```python
from build123d import *

# Parameters (mm, degrees)
SKETCH_2_R        = 9.874937623
EXTRUDE_1_DEPTH   = 40
SKETCH_2_R_2      = 10.181689967
EXTRUDE_1_2_DEPTH = 40
EXTRUDE_1_3_DEPTH = 40
EXTRUDE_5_DEPTH   = 40
EXTRUDE_2_DEPTH   = 4


# Read off the part's stored shape, not the designer's step: 拉伸-薄壁1
with BuildPart() as part:
    # 草图2 → Extrude 1 (new body)
    with BuildSketch(Plane(origin=(0, 140, 0), x_dir=(1, 0, 0), z_dir=(0, 1, 0))):
        with Locations(Location((-234.331213423, -10.749627478, 0), (0, 0, 270))):
            Circle(SKETCH_2_R)
    extrude_1 = extrude(amount=EXTRUDE_1_DEPTH)



with BuildPart() as body_2:
    # 草图2 → Extrude 1 2 (new body)
    with BuildSketch(Plane(origin=(0, 140, 0), x_dir=(1, 0, 0), z_dir=(0, 1, 0))):
        with Locations(Location((253.431386216, -10.749627478, 0), (0, 0, 270))):
            Circle(SKETCH_2_R_2)
    extrude_1_2 = extrude(amount=EXTRUDE_1_2_DEPTH)


with BuildPart() as part_1:
    add(part.part)

    add(body_2.part)  # Extrude 1 3 merges body 2
    # Extrude 1 3 outline → Extrude 1 3 (add)
    with BuildSketch(Plane.XY):
        with BuildLine():
            Line((-360, -135), (-350, -135))
            Line((-350, -135), (-335, -150))
            Line((-335, -150), (335, -150))
            ThreePointArc((335, -150), (345.606601718, -145.606601718), (350, -135))
            Line((350, -135), (350, 135))
            ThreePointArc((350, 135), (345.606601718, 145.606601718), (335, 150))
            Line((335, 150), (-335, 150))
            Line((-335, 150), (-335, 140))
            Line((-335, 140), (335, 140))
            ThreePointArc((335, 140), (338.535533906, 138.535533906), (340, 135))
            Line((340, 135), (340, -135))
            ThreePointArc((340, -135), (338.535533906, -138.535533906), (335, -140))
            Line((335, -140), (-330.857864376, -140))
            Line((-330.857864376, -140), (-341.617461171, -129.240403205))
            ThreePointArc((-341.617461171, -129.240403205), (-345.993586414, -118.835156387), (-350, -108.282039139))
            Line((-350, -108.282039139), (-350, 108.282039139))
            ThreePointArc((-350, 108.282039139), (-345.653254032, 119.682560505), (-340.875063682, 130.909090909))
            Line((-340.875063682, 130.909090909), (-350, 135))
            Line((-350, 135), (-360, 135))
            Line((-360, 135), (-360, 110.011554075))
            ThreePointArc((-360, 110.011554075), (-378.877101502, 0), (-360, -110.011554075))
            Line((-360, -110.011554075), (-360, -135))
        make_face()
        with BuildLine():
            Line((-360, 74.850130461), (-360, -74.850130461))
            ThreePointArc((-360, -74.850130461), (-368.877101502, 0), (-360, 74.850130461))
        make_face(mode=Mode.SUBTRACT)
    extrude(amount=EXTRUDE_1_3_DEPTH)

    # 镜向3: Extrude 1, Extrude 1 2 across plane
    add(extrude_1.mirror(Plane.ZX))
    add(extrude_1_2.mirror(Plane.ZX))

    # 草图1<3> → 拉伸-薄壁5 (add)
    with BuildSketch(Plane.XY):
        Polygon((-350, 135), (-335, 150), (-327.928932188, 142.928932188), (-342.928932188, 127.928932188), align=None)
    extrude(amount=EXTRUDE_5_DEPTH)

    # 草图1<4> → 凸台-拉伸2 (add)
    with BuildSketch(Plane.XY):
        with BuildLine():
            Line((-335, -150), (335, -150))
            ThreePointArc((335, -150), (345.606601718, -145.606601718), (350, -135))
            Line((350, -135), (350, 135))
            ThreePointArc((350, 135), (345.606601718, 145.606601718), (335, 150))
            Line((335, 150), (-335, 150))
            Line((-335, 150), (-350, 135))
            Line((-350, 135), (-350, -135))
            Line((-350, -135), (-335, -150))
        make_face()
    extrude(amount=EXTRUDE_2_DEPTH)


solid = part_1.part
```
For this review, take the finished solid that the model builds, in its own axes (mm). A direction names the side the tool comes from. Coordinates: 2 decimals unless noted, no trailing zeros. Order: outer loops, then holes, each group sorted by start corner. A loop starts at its lowest first (then second) coordinate and runs counter-clockwise, first axis right, second up. Notation, with made-up numbers: (76.5, -19.5) - (105.5, -19.5) arc R24 cw to (105.5, -5.5) - close; hole circle Ø5 at (-24.75, -2). An arc over 180 degrees is marked (long way). Answer as a JSON object with one key per item and string values. Group by question number.
1. We need section D-D on z = 10. Give the number of separate pieces and of enclosed holes in the cut face, then the cut area to 3 significant figures.
2. We need section A-A on y = 18. State the section outline as (x, z) points.
3. The part is to be moulded in two halves that separate along Y. For faces 4 (the flat face through (-10, 2, 4)), 5 (the cylindrical face through (243.5, 164.8, 8.5)), 6 (the flat face through (-343, -142, 20)), say which applies: pulls with the +Y half, pulls with the -Y half, needs draft (parallel to the pull), parting line crosses it, or undercut.
4. We need section C-C on y = -67. State the section outline as (x, z) points.
5. We need section B-B on x = -101. State the section outline as (y, z) points, then the cut area to 3 significant figures.
6. Clearance check with flat-ended pins moving along their axes: P1, Ø8, axis at x = -356.5, z = 26, coming from the -Y side; P2, Ø5, axis at x = 241.5, y = -123.5, coming from the +Z side; P3, Ø18, axis at x = 50, z = 31, coming from the +Y side; P4, Ø4, axis at x = 29, y = 120, coming from the -Z side. State where each tip first meets the part, or that it passes through.
7. For faces 1 (the cylindrical face through (-243.97, -164.79, 8.61)), 2 (the cylindrical face through (-345.935, -118.982, 21.748)), 3 (the flat face through (254, -180, 11)), list the 3-axis set-ups (+Z, -Z, +X, -X, +Y, -Y) from which the entire face can be reached by the end or side of a thin tool; tool diameter is ignored.
8. For probe 1 along X at (y, z) = (80, 20.5); probe 2 along Y at (x, z) = (-64, 14); probe 3 along X at (y, z) = (-56.5, 20), list the stretches that pass through material, from the lowest coordinate up.
Final values:
{
 "1": {"separate pieces": "1", "enclosed holes": "2", "area": "24,000 mm²"},
 "2": {"outline": "(-378.39, 0) - (-368.37, 0) - (-368.37, 40) - (-378.39, 40) - close; (-360, 0) - (350, 0) - (350, 40) - (340, 40) - (340, 4) - (-350, 4) - (-350, 40) - (-360, 40) - close"},
 "3": {"face 4": "undercut", "face 5": "needs draft", "face 6": "pulls with the -Y half"},
 "4": {"outline": "(-372, 0) - (-361.78, 0) - (-361.78, 40) - (-372, 40) - close; (-360, 0) - (350, 0) - (350, 40) - (340, 40) - (340, 4) - (-350, 4) - (-350, 40) - (-360, 40) - close"},
 "5": {"outline": "(-150, 0) - (150, 0) - (150, 40) - (140, 40) - (140, 4) - (-140, 4) - (-140, 40) - (-150, 40) - close", "area": "1,920 mm²"},
 "6": {"P1": "y = -135", "P2": "z = 4", "P3": "y = 150", "P4": "z = 0"},
 "7": {"face 1": "-Y", "face 2": "+Z", "face 3": "+Z, -Z, +X, -X, -Y"},
 "8": {"probe 1": "-369.03 to -350, 340 to 350", "probe 2": "-150 to -140, 140 to 150", "probe 3": "-374 to -363.85, -360 to -350, 340 to 350"}
}
